CAD build for the part. Positions are in the model's coordinates, mm. Round coordinates to 2 decimals unless told otherwise and drop trailing zeros. Loops run counter-clockwise (first coordinate to the right, second up) from the corner with the lowest first, then second, coordinate; pieces in that order, holes last. Notation, with made-up numbers: (18, 75.5) -> (42, 75.5) arc R15 ccw to (42, 88.5) -> close; hole circle Ø7 at (20.25, 71). An arc over 180 degrees is marked (long way). Answer as CSV lines item,"result".
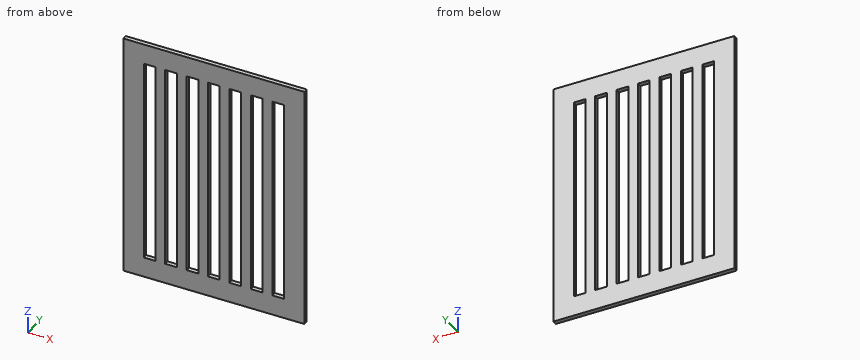
```python
from build123d import *

# Parameters (mm, degrees)
F0_W     = 785
F0_H     = 1078
F0_W_2   = 607
F0_H_2   = 900
F1_DEPTH = 19
F2_W     = 42
F2_H     = 19
F3_DEPTH = 900


with BuildPart() as f1:
    # F0 (on Front) → F1 (new body)
    with BuildSketch(Plane.XZ):
        Rectangle(F0_W, F0_H)
        Rectangle(F0_W_2, F0_H_2, mode=Mode.SUBTRACT)
    extrude(amount=F1_DEPTH)

    # F2 (on face) → F3 (join, through all)
    with BuildSketch(Plane(origin=(0, 0, 450), x_dir=(1, 0, 0), z_dir=(0, 0, -1))):
        with Locations((-232.5, 9.5)):
            Rectangle(F2_W, F2_H)
        with Locations((-139.5, 9.5)):
            Rectangle(F2_W, F2_H)
        with Locations((-46.5, 9.5)):
            Rectangle(F2_W, F2_H)
        with Locations((46.5, 9.5)):
            Rectangle(F2_W, F2_H)
        with Locations((139.5, 9.5)):
            Rectangle(F2_W, F2_H)
        with Locations((232.5, 9.5)):
            Rectangle(F2_W, F2_H)
    extrude(amount=F3_DEPTH)


solid = f1.part
```
Q1. Slice it at A-A, the plane z = 326. Count the separate pieces of the cut face and the enclosed holes in it, and give its area (3 significant figures).
Results:
separate pieces,"8"
enclosed holes,"0"
area,"8,170 mm2"
Q2. Slice it at B-B, the plane x = -1. Give the cut face in (y, z).
Results:
outline,"(-19, -539) -> (0, -539) -> (0, -450) -> (-19, -450) -> close; (-19, 450) -> (0, 450) -> (0, 539) -> (-19, 539) -> close"
Q3. Probe L1, parallel to Z at x = 265, y = -14.5. List the from-to ranges inside material, lowest first. Write a range as [from, to].
Results:
L1,"[-539, -450], [450, 539]"
